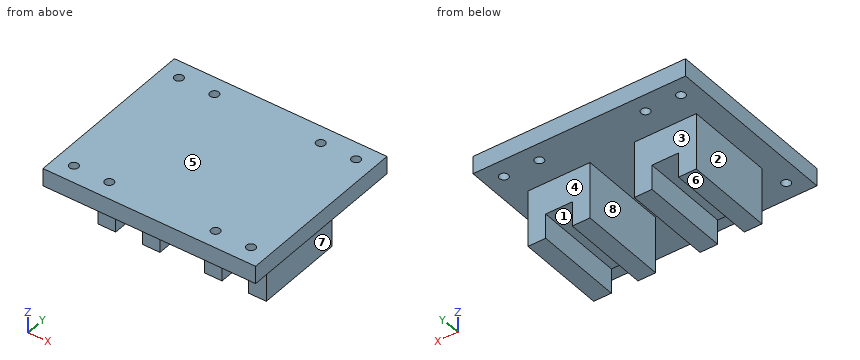
```python
from build123d import *

# Parameters (mm, degrees)
SKETCH_W     = 120
SKETCH_H     = 100
SKETCH_R     = 2.5
PAD_DEPTH    = 10
SKETCH001_W  = 35
SKETCH001_H  = 50
PAD001_DEPTH = 18
SKETCH002_W  = 10
SKETCH002_H  = 50
PAD002_DEPTH = 14


with BuildPart() as part:
    # Sketch → Pad (new body)
    with BuildSketch(Plane.XY):
        Rectangle(SKETCH_W, SKETCH_H)
        with Locations((-50, 40)):
            Circle(SKETCH_R, mode=Mode.SUBTRACT)
        with Locations((-30, 40)):
            Circle(SKETCH_R, mode=Mode.SUBTRACT)
        with Locations((30, 40)):
            Circle(SKETCH_R, mode=Mode.SUBTRACT)
        with Locations((50, 40)):
            Circle(SKETCH_R, mode=Mode.SUBTRACT)
        with Locations((-50, -40)):
            Circle(SKETCH_R, mode=Mode.SUBTRACT)
        with Locations((-30, -40)):
            Circle(SKETCH_R, mode=Mode.SUBTRACT)
        with Locations((30, -40)):
            Circle(SKETCH_R, mode=Mode.SUBTRACT)
        with Locations((50, -40)):
            Circle(SKETCH_R, mode=Mode.SUBTRACT)
    extrude(amount=PAD_DEPTH)

    # Sketch001 (on Face13 of Pad) → Pad001 (join)
    with BuildSketch(Plane(origin=(0, 0, 0), x_dir=(1, 0, 0), z_dir=(0, 0, -1))):
        with Locations((-30, 0)):
            Rectangle(SKETCH001_W, SKETCH001_H)
        with Locations((30, 0)):
            Rectangle(SKETCH001_W, SKETCH001_H)
    extrude(amount=PAD001_DEPTH)

    # Sketch002 (on Face23 of Pad001) → Pad002 (join)
    with BuildSketch(Plane(origin=(0, 0, -18), x_dir=(1, 0, 0), z_dir=(0, 0, -1))):
        with Locations((-42.5, 0)):
            Rectangle(SKETCH002_W, SKETCH002_H)
        with Locations((-17.5, 0)):
            Rectangle(SKETCH002_W, SKETCH002_H)
        with Locations((17.5, 0)):
            Rectangle(SKETCH002_W, SKETCH002_H)
        with Locations((42.5, 0)):
            Rectangle(SKETCH002_W, SKETCH002_H)
    extrude(amount=PAD002_DEPTH)


solid = part.part
```
For this review, take the finished solid that the model builds, in its own axes (mm). Face numbers are marked on the shaded views. A direction names the side the tool comes from. Round coordinates to 2 decimals unless told otherwise and drop trailing zeros. Write each loop counter-clockwise with the first axis right and the second up, starting at its lowest first coordinate (ties: lowest second). Pieces come first, ordered by that corner, then holes. Notation, with made-up numbers: (1, 55.25) -> (11, 55.25) arc R31 cw to (11, 84.25) -> close; hole circle Ø1 at (6, -23.5). An arc over 180 degrees is marked (long way). Use one line per item in the form item = value.
Q1. Consider section C-C (z = -24). State the section outline as (x, y) points.
Resolved:
outline = (-47.5, -25) -> (-37.5, -25) -> (-37.5, 25) -> (-47.5, 25) -> close; (-22.5, -25) -> (-12.5, -25) -> (-12.5, 25) -> (-22.5, 25) -> close; (12.5, -25) -> (22.5, -25) -> (22.5, 25) -> (12.5, 25) -> close; (37.5, -25) -> (47.5, -25) -> (47.5, 25) -> (37.5, 25) -> close
Q2. Consider section B-B (x = 30). State the section outline as (y, z) points.
Resolved:
outline = (-50, 0) -> (-42.5, 0) -> (-42.5, 10) -> (-50, 10) -> close; (-37.5, 0) -> (-25, 0) -> (-25, -18) -> (25, -18) -> (25, 0) -> (37.5, 0) -> (37.5, 10) -> (-37.5, 10) -> close; (42.5, 0) -> (50, 0) -> (50, 10) -> (42.5, 10) -> close
Q3. To check wall thickness, follow probe 1 along Y at (x, z) = (50, 4); probe 2 along X at (y, z) = (17.5, -16); probe 3 along Z at (x, y) = (36, 5.5). State the ranges of each line that lie inside material, in increasing order. Write a range as from..to.
Resolved:
probe_1 = -50..-42.5, -37.5..37.5, 42.5..50
probe_2 = -47.5..-12.5, 12.5..47.5
probe_3 = -18..10
Q4. The part is to be moulded in two halves that separate along X. For the marked faces 1, 2 and 3, say which applies: released by +X, released by -X, zero draft, split by the parting line, or undercut.
Resolved:
face_1 = undercut
face_2 = released by -X
face_3 = zero draft
Q5. Machinability: for the marked faces 4, 5, 6, 7 and 8, which of the approach directions +Z, -Z, +X, -X, +Y, -Y give a long, thin tool a straight path to every point of the face, cutting with its end or side? Answer none if there is none.
Resolved:
face_4 = -Z, +X, -X, +Y
face_5 = +Z, +X, -X, +Y, -Y
face_6 = -Z, +X, -X, +Y, -Y
face_7 = -Z, +X, +Y, -Y
face_8 = -Z, +Y, -Y
Q6. Clearance check with flat-ended pins moving along their axes: pin 1 Ø3 at (x, y) = (-50, -40) entering from +Z; pin 2 Ø5 at (x, y) = (30.5, -2) entering from -Z; pin 3 Ø7 at (y, z) = (-6.5, -25.5) entering from -X; pin 4 Ø4 at (y, z) = (-2, -23.5) entering from +X. State where each tip first meets the part, or that it passes through.
Resolved:
pin_1 = through
pin_2 = -18
pin_3 = -47.5
pin_4 = 47.5
Q7. Consider section D-D (y = -40). State the section outline as (x, z) points, then the cut area to 3 significant figures.
Resolved:
outline = (-60, 0) -> (-52.5, 0) -> (-52.5, 10) -> (-60, 10) -> close; (-47.5, 0) -> (-32.5, 0) -> (-32.5, 10) -> (-47.5, 10) -> close; (-27.5, 0) -> (27.5, 0) -> (27.5, 10) -> (-27.5, 10) -> close; (32.5, 0) -> (47.5, 0) -> (47.5, 10) -> (32.5, 10) -> close; (52.5, 0) -> (60, 0) -> (60, 10) -> (52.5, 10) -> close
area = 1,000 mm²
Q8. Consider section A-A (z = -3). State the section outline as (x, y) points, then the cut area to 3 significant figures.
Resolved:
outline = (-47.5, -25) -> (-12.5, -25) -> (-12.5, 25) -> (-47.5, 25) -> close; (12.5, -25) -> (47.5, -25) -> (47.5, 25) -> (12.5, 25) -> close
area = 3,500 mm²
